For this review, take the finished solid that the model builds, in its own axes (mm). Face numbers are marked on the shaded views. A direction names the side the tool comes from. Round coordinates to 2 decimals unless told otherwise and drop trailing zeros. Loops run counter-clockwise (first coordinate to the right, second up) from the corner with the lowest first, then second, coordinate; pieces in that order, holes last.
```python
from build123d import *

# Parameters (mm, degrees)
SKETCH1_R           = 60
BOSS_EXTRUDE1_DEPTH = 30
SKETCH2_R           = 10
CUT_EXTRUDE1_DEPTH  = 180.223980285


with BuildPart() as part:
    # Sketch1 → Boss-Extrude1 (new body)
    with BuildSketch(Plane(origin=(0, 0, 0), x_dir=(0, 0, -1), z_dir=(1, 0, 0))):
        with BuildLine():
            Line((114.414215067, -60), (44.414215067, -60))
            ThreePointArc((44.414215067, -60), (0, 74.65), (-44.414215067, -60))
            Line((-44.414215067, -60), (-114.414215067, -60))
            Line((-114.414215067, -60), (-114.414215067, -84.8))
            Line((-114.414215067, -84.8), (114.414215067, -84.8))
            Line((114.414215067, -84.8), (114.414215067, -60))
        make_face()
        Circle(SKETCH1_R, mode=Mode.SUBTRACT)
    extrude(amount=BOSS_EXTRUDE1_DEPTH)

    # Sketch2 → Cut-Extrude1 (cut, through all)
    with BuildSketch(Plane(origin=(0, -60, 0), x_dir=(1, 0, 0), z_dir=(0, 1, 0))):
        with Locations(Location((15, -94.532107533, 0), (0, 0, 270))):
            Circle(SKETCH2_R)
        with Locations(Location((15, 94.532107533, 0), (0, 0, 270))):
            Circle(SKETCH2_R)
    extrude(amount=-CUT_EXTRUDE1_DEPTH, mode=Mode.SUBTRACT)


solid = part.part
```
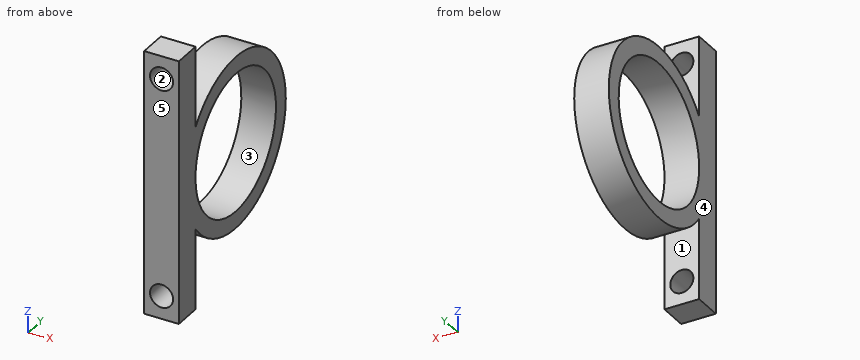
(1) Add section D-D (y = 64). Give the boundary of the cut face in (x, z), plus the area to 3 significant figures.
(2) For the marked faces 1 and 2, list the 3-axis set-ups (+Z, -Z, +X, -X, +Y, -Y) from which the entire face can be reached by the end or side of a thin tool; tool diameter is ignored.
(3) Insertion check: pin 1 Ø18 at (x, z) = (15, 94.53) entering from +Y; pin 2 Ø4 at (x, y) = (26, -3) entering from -Z; pin 3 Ø8 at (x, y) = (24.5, -35) entering from -Z; pin 4 Ø9 at (x, z) = (21, -63) entering from +Y. Each pin has a flat end and moves straight along its axis. Give the tip position at first contact, or say it passes through.
(4) The part is to be moulded in two halves that separate along Y. For the marked faces 3, 4 and 5, say which applies: pulls with the +Y half, pulls with the -Y half, needs draft (parallel to the pull), parting line crosses it, or undercut.
(5) For L1, parallel to Z at x = 14, y = -63; L2, parallel to Y at x = 12.75, z = -50; L3, parallel to Y at x = 16.5, z = 52, list the stretches that pass through material, from the lowest coordinate up.
(6) Add section B-B (y = 0). Give the boundary of the cut face in (x, z), plus the area to 3 significant figures.
(7) Add section A-A (x = 15). Give the boundary of the cut face in (y, z).
(8) Add section C-C (z = 0). Give the boundary of the cut face in (x, y).
Outcome:
1. outline: (0, -38.43) - (30, -38.43) - (30, 38.43) - (0, 38.43) - close
1. area: 2,310 mm2
2. face 1: -Z, +X, -X
2. face 2: +Y, -Y
3. pin 1: passes through
3. pin 2: stops at z = -74.64
3. pin 3: stops at z = -67.91
3. pin 4: stops at y = 46.37
4. face 3: undercut
4. face 4: needs draft
4. face 5: pulls with the -Y half
5. L1: z = -114.41 to -104.48, -84.58 to 84.58, 104.48 to 114.41
5. L2: y = -84.8 to -60, -55.43 to -33.17, 33.17 to 55.43
5. L3: y = -84.8 to -60, -53.56 to -29.93, 29.93 to 53.56
6. outline: (0, -74.65) - (30, -74.65) - (30, -60) - (0, -60) - close; (0, 60) - (30, 60) - (30, 74.65) - (0, 74.65) - close
6. area: 879 mm2
7. outline: (-84.8, -114.41) - (-60, -114.41) - (-60, -104.53) - (-84.8, -104.53) - close; (-84.8, -84.53) - (-60, -84.53) - (-60, -44.41) arc R74.65 ccw (long way) to (-60, 44.41) - (-60, 84.53) - (-84.8, 84.53) - close; (-84.8, 104.53) - (-60, 104.53) - (-60, 114.41) - (-84.8, 114.41) - close; hole circle Ø120 at (0, 0)
8. outline: (0, -84.8) - (30, -84.8) - (30, -60) - (0, -60) - close; (0, 60) - (30, 60) - (30, 74.65) - (0, 74.65) - close
